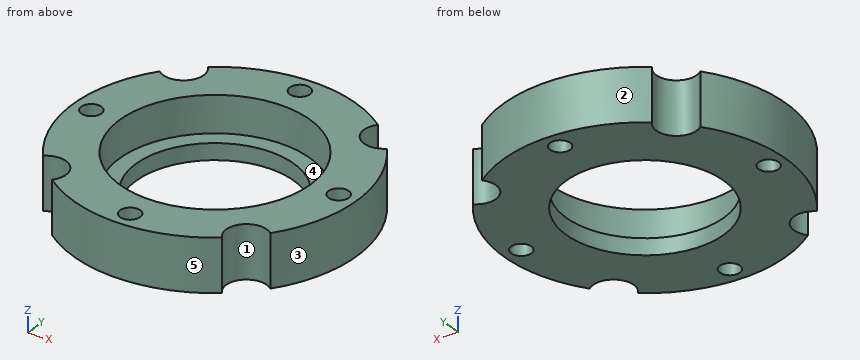
from build123d import *

# Parameters (mm, degrees)
SZKIC1_R                    = 35
SZKIC1_R_2                  = 30.5
SZKIC1_R_3                  = 19.5
DODANIE_WYCI_GNI_CIE1_DEPTH = 13
OTWORY_USTALAJ_CE_5_0MM1_D  = 5
WYTNIJ_WYCI_GNI_CIE1_START  = -9
SZKIC6_R                    = 23.5
SZKIC6_R_2                  = 19.5
WYTNIJ_WYCI_GNI_CIE1_DEPTH  = 9
SZKIC2_R                    = 5
WYTNIJ_WYCI_GNI_CIE2_DEPTH  = 14


with BuildPart() as part:
    # Szkic1 → Dodanie-wyciągnięcie1 (new body)
    # profile 1 of 2: a face of its own
    with BuildSketch(Plane.XY):
        with Locations(Location((0, 0, 0), (0, 0, 180))):
            Circle(SZKIC1_R)
        Circle(SZKIC1_R_2, mode=Mode.SUBTRACT)
    # profile 2 of 2: a face of its own
    with BuildSketch(Plane.XY):
        Circle(SZKIC1_R_2)
        with Locations(Location((0, 0, 0), (0, 0, 180))):
            Circle(SZKIC1_R_3, mode=Mode.SUBTRACT)
    extrude(amount=DODANIE_WYCI_GNI_CIE1_DEPTH)

    # Otwory ustalające Ø5.0mm1 (through all)
    with Locations(Plane.XY.offset(13)):
        with Locations((0, 30.5), (0, -30.5), (-30.5, 0), (30.5, 0)):
            Hole(OTWORY_USTALAJ_CE_5_0MM1_D / 2)

    # Szkic6 → Wytnij-wyciągnięcie1 (cut)
    with BuildSketch(Plane.XY.offset(13).offset(WYTNIJ_WYCI_GNI_CIE1_START)):
        Circle(SZKIC6_R)
        with Locations(Location((0, 0, 0), (0, 0, 180))):
            Circle(SZKIC6_R_2, mode=Mode.SUBTRACT)
    extrude(amount=WYTNIJ_WYCI_GNI_CIE1_DEPTH, mode=Mode.SUBTRACT)

    # Szkic2 → Wytnij-wyciągnięcie2 (cut)
    with BuildSketch(Plane.XY.offset(13)):
        with Locations((24.748737342, 24.748737342)):
            Circle(SZKIC2_R)
        with Locations((24.748737342, -24.748737342)):
            Circle(SZKIC2_R)
        with Locations((-24.748737342, -24.748737342)):
            Circle(SZKIC2_R)
        with Locations((-24.748737342, 24.748737342)):
            Circle(SZKIC2_R)
    extrude(amount=-WYTNIJ_WYCI_GNI_CIE2_DEPTH, mode=Mode.SUBTRACT)


solid = part.part
Input: part model. Units: mm. Frame: model coordinates. Face numbers are marked on the shaded views. A direction names the side the tool comes from. Round coordinates to 2 decimals unless told otherwise and drop trailing zeros. Order: outer loops, then holes, each group sorted by start corner. A loop starts at its lowest first (then second) coordinate and runs counter-clockwise, first axis right, second up. Notation, with made-up numbers: (74.25, 10) - (82.25, 10) arc R13 cw to (82.25, 28) - close; hole circle Ø3 at (64.25, 58.25). An arc over 180 degrees is marked (long way). Answer as a JSON object with one key per item and string values. Group by question number.
(1) Draft query along Y for the marked faces 1, 2 and 3. Return one class per face: released by +Y, released by -Y, zero draft, split by the parting line, or undercut.
(2) Cut plane C-C (z = 1.25). Return loops of the section in (x, y), then the cut area to 3 significant figures.
(3) Cut plane D-D (y = -8). Return loops of the section in (x, z).
(4) Material intervals for probe 1 along Y at (x, z) = (0, 3.25); probe 2 along Y at (x, z) = (0, 6); probe 3 along X at (y, z) = (2, 8.25), sorted ascending. Write a range as from..to.
(5) Reachability of the marked faces 4 and 5 from +Z, -Z, +X, -X, +Y, -Y: full face, straight path, thin tool, end or side. Return the list, or none.
(6) Pin query (flat end, axial travel): P1, Ø4.5, axis at x = -30.5, y = 0, coming from the +Z side; P2, Ø5, axis at x = 11.5, y = 17, coming from the +Z side; P3, Ø1.5, axis at x = 7, z = 11, coming from the +Y side; P4, Ø1.5, axis at x = 8.5, z = 2.5, coming from the -Y side. Return the tip coordinate at first contact, or that it passes through.
(7) Cut plane A-A (x = 0). Return loops of the section in (y, z).
Here are the results:
{
 "1": {"face 1": "undercut", "face 2": "released by +Y", "face 3": "split by the parting line"},
 "2": {"outline": "(-28.02, -20.97) arc R5 cw to (-20.97, -28.02) arc R35 ccw to (20.97, -28.02) arc R5 cw to (28.02, -20.97) arc R35 ccw to (28.02, 20.97) arc R5 cw to (20.97, 28.02) arc R35 ccw to (-20.97, 28.02) arc R5 cw to (-28.02, 20.97) arc R35 ccw to start; hole circle Ø5 at (-30.5, 0); hole circle Ø39 at (0, 0); hole circle Ø5 at (0, -30.5); hole circle Ø5 at (0, 30.5); hole circle Ø5 at (30.5, 0)", "area": "2,420 mm^2"},
 "3": {"outline": "(-34.07, 0) - (-17.78, 0) - (-17.78, 4) - (-22.1, 4) - (-22.1, 13) - (-34.07, 13) - close; (17.78, 0) - (34.07, 0) - (34.07, 13) - (22.1, 13) - (22.1, 4) - (17.78, 4) - close"},
 "4": {"probe 1": "y = -35..-33, -28..-19.5, 19.5..28, 33..35", "probe 2": "y = -35..-33, -28..-23.5, 23.5..28, 33..35", "probe 3": "x = -34.94..-32, -29..-23.41, 23.41..29, 32..34.94"},
 "5": {"face 4": "+Z", "face 5": "+Z, -Z, -Y"},
 "6": {"P1": "passes through", "P2": "stops at z = 4", "P3": "stops at y = 34.44", "P4": "stops at y = -34.13"},
 "7": {"outline": "(-35, 0) - (-33, 0) - (-33, 13) - (-35, 13) - close; (-28, 0) - (-19.5, 0) - (-19.5, 4) - (-23.5, 4) - (-23.5, 13) - (-28, 13) - close; (19.5, 0) - (28, 0) - (28, 13) - (23.5, 13) - (23.5, 4) - (19.5, 4) - close; (33, 0) - (35, 0) - (35, 13) - (33, 13) - close"}
}
